```python
from build123d import *

# Parameters (mm, degrees)
SKETCH_2_R        = 11
SKETCH_2_R_2      = 1.5
EXTRUDE_483_DEPTH = 4
SKETCH_3_W        = 18
SKETCH_3_H        = 26.8
EXTRUDE_726_DEPTH = 4
EXTRUDE_922_DEPTH = 2


with BuildPart() as part:
    # Эскиз2 → Extrude 483 (new body)
    with BuildSketch(Plane(origin=(0, 0, 0), x_dir=(1, 0, 0), z_dir=(0, 1, 0))):
        with BuildLine():
            Line((-15.5, -20.5), (15.5, -20.5))
            ThreePointArc((15.5, -20.5), (19.035533906, -19.035533906), (20.5, -15.5))
            Line((20.5, -15.5), (20.5, 15.5))
            ThreePointArc((20.5, 15.5), (19.035533906, 19.035533906), (15.5, 20.5))
            Line((15.5, 20.5), (-15.5, 20.5))
            ThreePointArc((-15.5, 20.5), (-19.035533906, 19.035533906), (-20.5, 15.5))
            Line((-20.5, 15.5), (-20.5, -15.5))
            ThreePointArc((-20.5, -15.5), (-19.035533906, -19.035533906), (-15.5, -20.5))
        make_face()
        with Locations(Location((0, 0, 0), (0, 0, 270))):
            Circle(SKETCH_2_R, mode=Mode.SUBTRACT)
        with Locations(Location((-15.5, 15.5, 0), (0, 0, 270))):
            Circle(SKETCH_2_R_2, mode=Mode.SUBTRACT)
        with Locations(Location((15.5, -15.5, 0), (0, 0, 90))):
            Circle(SKETCH_2_R_2, mode=Mode.SUBTRACT)
        with Locations(Location((-15.5, -15.5, 0), (0, 0, 90))):
            Circle(SKETCH_2_R_2, mode=Mode.SUBTRACT)
        with Locations(Location((15.5, 15.5, 0), (0, 0, 270))):
            Circle(SKETCH_2_R_2, mode=Mode.SUBTRACT)
    extrude(amount=EXTRUDE_483_DEPTH)

    # Эскиз3 → Extrude 726 (add)
    with BuildSketch(Plane.XY.offset(20.5)):
        with Locations((0, -9.4)):
            Rectangle(SKETCH_3_W, SKETCH_3_H)
    extrude(amount=EXTRUDE_726_DEPTH)

    # Эскиз4 → Extrude 922 (add)
    with BuildSketch(Plane.XZ.offset(22.8)):
        with BuildLine():
            Line((9, 24.5), (-9, 24.5))
            Line((-9, 24.5), (-9, 32.5))
            ThreePointArc((-9, 32.5), (-7.242640687, 36.742640687), (-3, 38.5))
            Line((-3, 38.5), (3, 38.5))
            ThreePointArc((3, 38.5), (7.242640687, 36.742640687), (9, 32.5))
            Line((9, 32.5), (9, 24.5))
        make_face()
    extrude(amount=-EXTRUDE_922_DEPTH)


solid = part.part
```
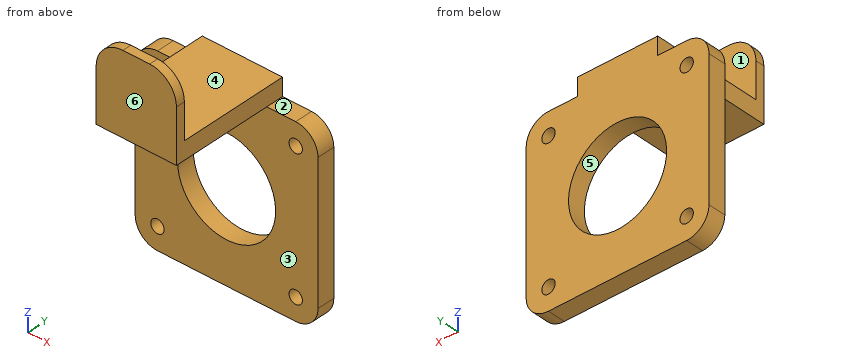
Work out the finished part from the listing and answer in its coordinate system (mm). Face numbers are marked on the shaded views. A direction names the side the tool comes from. Give positions to 0.01 mm unless a question says otherwise; leave off trailing zeros. Loops run counter-clockwise (first coordinate to the right, second up) from the corner with the lowest first, then second, coordinate; pieces in that order, holes last. Notation, with made-up numbers: (74.5, 54.5) -> (130.5, 54.5) arc R25 cw to (130.5, 67.5) -> close; hole circle Ø6 at (34, 78). An arc over 180 degrees is marked (long way). Write item = value, one per line. Start each with the question number.
(1) Given pin 1 Ø12.5 at (x, z) = (-7.5, 6.5) entering from -Y; pin 2 Ø12 at (x, y) = (10.5, -18.5) entering from -Z; pin 3 Ø13 at (y, z) = (-6.5, 28.5) entering from -X, each flat-ended and moving along its own axis, determine where each tip first touches the part or whether it passes through.
(2) Find the intervals of material crossed by probe 1 along X at (y, z) = (1, 15.5); probe 2 along X at (y, z) = (1.8, 0); probe 3 along Z at (x, y) = (16, 1.25), in increasing order. Write a range as from..to.
(3) Find section A-A on z = 0. Give the vertices of the cut face in (x, y).
(4) Find section C-C on x = 0. Give the vertices of the cut face in (y, z), and give its area (3 significant figures).
(5) The mould has two halves that part along Z. Classify the marked faces 4, 5 and 6: +Z half, -Z half, draft (parallel to the pull), parting line (faces both ways), or undercut.
(6) Find section B-B on x = 5. Give the vertices of the cut face in (y, z), and give its area (3 significant figures).
(7) Find section D-D on z = 7. Give the vertices of the cut face in (x, y), and give its area (3 significant figures).
(8) Which of the six approach directions +Z, -Z, +X, -X, +Y, -Y give full straight-line access (tool end or side, diameter ignored) to the marked faces 1, 2 and 3?
From the geometry:
q1.pin_1 = 0
q1.pin_2 = 20.5
q1.pin_3 = -9
q2.probe_1 = -20.5..-17, -14..14, 17..20.5
q2.probe_2 = -20.5..-11, 11..20.5
q2.probe_3 = -20.47..-16.91, -14.09..14.09, 16.91..20.47
q3.outline = (-20.5, 0) -> (-11, 0) -> (-11, 4) -> (-20.5, 4) -> close; (11, 0) -> (20.5, 0) -> (20.5, 4) -> (11, 4) -> close
q4.outline = (-22.8, 20.5) -> (0, 20.5) -> (0, 11) -> (4, 11) -> (4, 24.5) -> (-20.8, 24.5) -> (-20.8, 38.5) -> (-22.8, 38.5) -> close; (0, -20.5) -> (4, -20.5) -> (4, -11) -> (0, -11) -> close
q4.area = 211 mm^2
q5.face_4 = +Z half
q5.face_5 = undercut
q5.face_6 = draft
q6.outline = (-22.8, 20.5) -> (0, 20.5) -> (0, 9.8) -> (4, 9.8) -> (4, 24.5) -> (-20.8, 24.5) -> (-20.8, 38.16) -> (-22.8, 38.16) -> close; (0, -20.5) -> (4, -20.5) -> (4, -9.8) -> (0, -9.8) -> close
q6.area = 220 mm^2
q7.outline = (-20.5, 0) -> (-8.49, 0) -> (-8.49, 4) -> (-20.5, 4) -> close; (8.49, 0) -> (20.5, 0) -> (20.5, 4) -> (8.49, 4) -> close
q7.area = 96.1 mm^2
q8.face_1 = +Z, +X, -X, +Y
q8.face_2 = +Z, +X, +Y, -Y
q8.face_3 = -Z, +X, -X, -Y
